```python
from build123d import *

# Parameters (mm, degrees)
F0_W    = 1
F0_H    = 1
F2_SIZE = 0.99999
F5_R    = 2


# Not quite as in the source:
# - a fillet or chamfer is up to 0.001 mm smaller than in the source, because OpenCascade refuses the exact size


with BuildPart() as f1:
    # F0 (on Top) → F1 (revolve)
    with BuildSketch(Plane.XY):
        Polygon((0, 21), (0, 0), (11.5, 0), (11.5, 2), (11.5, 3), (11.5, 6), (11.5, 7), (11.5, 10), (11.5, 11), (11.5, 14), (11.5, 15), (11.5, 18), (14.5, 18), (14.5, 21), align=None)
        with Locations((12, 14.5)):
            Rectangle(F0_W, F0_H)
        with Locations((12, 10.5)):
            Rectangle(F0_W, F0_H)
        with Locations((12, 6.5)):
            Rectangle(F0_W, F0_H)
        with Locations((12, 2.5)):
            Rectangle(F0_W, F0_H)
    revolve(axis=Axis((0, 10.5, 0), (0, 1, 0)))

    # F2 (size 1 in the source; OpenCascade refuses exactly that, so slightly less here)
    f2_edges = [f1.edges().sort_by_distance(p)[0] for p in [
        (-11.5, 2, 0),
        (-11.5, 6, 0),
        (-11.5, 10, 0),
        (-11.5, 14, 0),
    ]]
    chamfer(f2_edges, length=F2_SIZE)

    # F3 (on Top) → F4 (revolve)
    with BuildSketch(Plane.XY):
        with BuildLine():
            ThreePointArc((0, 18.5), (8.8388347648, 22.1611652352), (12.5, 31))
            ThreePointArc((12.5, 31), (8.8388347648, 39.8388347648), (0, 43.5))
            Line((0, 43.5), (0, 18.5))
        make_face()
    revolve(axis=Axis((0, 31, 0), (0, -1, 0)))

    # F5
    f5_edges = [f1.edges().sort_by_distance(p)[0] for p in [
        (-7.5, 21, 0),
    ]]
    fillet(f5_edges, radius=F5_R)


solid = f1.part
```
The model under review builds one solid part; all positions refer to its coordinate system, in mm. A direction names the side the tool comes from. Round coordinates to 2 decimals unless told otherwise and drop trailing zeros. Write each loop counter-clockwise with the first axis right and the second up, starting at its lowest first coordinate (ties: lowest second). Pieces come first, ordered by that corner, then holes. Notation, with made-up numbers: (57.25, -32.5) - (63.25, -32.5) arc R31 ccw to (63.25, -0.5) - close; hole circle Ø7 at (55, -1.75). An arc over 180 degrees is marked (long way). Use one line per item in the form item = value.
Q1. Consider section B-B (y = 4). State the section outline as (x, z) points, and give its area (3 significant figures).
Answer key:
outline = circle Ø23 at (0, 0)
area = 415 mm2
Q2. For line 1 (Y direction, x = 11.5, z = 1); line 2 (Y direction, x = -11.25, z = 0); line 3 (Y direction, x = -8, z = -9.75), list the stretches that pass through material, from the lowest coordinate up. Write a range as [from, to].
Answer key:
line_1 = [1.04, 3], [5.04, 7], [9.04, 11], [13.04, 15], [18, 21.08], [26.2, 35.8]
line_2 = [0, 21.19], [25.55, 36.45]
line_3 = [18, 21]
Q3. Consider section A-A (y = 9.5). State the section outline as (x, z) points.
Answer key:
outline = circle Ø24 at (0, 0)
Q4. Insertion check: pin 1 Ø8 at (x, z) = (-11.5, -5.5) entering from +Y; pin 2 Ø6 at (y, z) = (31, -11) entering from -X; pin 3 Ø12 at (y, z) = (22.5, 7) entering from -X. Each pin has a flat end and moves straight along its axis. Give the tip position at first contact, or say it passes through.
Answer key:
pin_1 = 39.93
pin_2 = -9.6
pin_3 = -14.45
Q5. Tool access review of faces 4 (the cylindrical face through (11.923, 2.507, -3.755)), 5 (the flat face through (3, 21, 12)): name each direction out of +Z, -Z, +X, -X, +Y, -Y from which nothing blocks a thin tool from reaching the whole face with its end or side.
Answer key:
face_4 = -Y
face_5 = none
Q6. Draft analysis for pull direction Y (two halves, no side actions). For faces 1 (the cylindrical face through (6.691, 19.521, 12.864)), 2 (the flat face through (0, 0, 0)), 3 (the flat face through (-11, 3, 4)), state which applies: +Y half, -Y half, draft (parallel to the pull), parting line (faces both ways), or undercut.
Answer key:
face_1 = draft
face_2 = -Y half
face_3 = undercut
